from build123d import *

# Parameters (mm, degrees)
F0_R     = 77.1800342887
F0_R_2   = 66.4755295027
F1_DEPTH = 25.4
F2_DEPTH = 25.4
F3_DEPTH = 67.056


with BuildPart() as f1:
    # F0 (on Top) → F1 (new body)
    with BuildSketch(Plane.XY):
        Circle(F0_R)
        Circle(F0_R_2, mode=Mode.SUBTRACT)
    extrude(amount=F1_DEPTH)

    # F2 (add): faces of the model
    f2_faces = [f1.faces().sort_by_distance(p)[0] for p in [
        (-74.997053264, 0, 0),
        (-74.997053264, 0, 25.4),
    ]]
    extrude(f2_faces, amount=F2_DEPTH, dir=(0, 0, -1))

    # F3 (add): a face of the model
    f3_faces = [f1.faces().sort_by_distance(p)[0] for p in [
        (-74.997053264, 0, 25.4),
    ]]
    extrude(f3_faces, amount=F3_DEPTH)


solid = f1.part
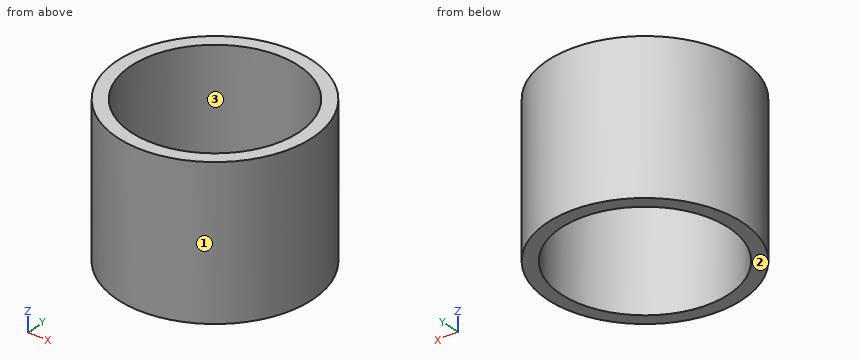
Design review of the part built by this model. Coordinates are the model's own, in mm. Face numbers are marked on the shaded views. Coordinates: 2 decimals unless noted, no trailing zeros. Order: outer loops, then holes, each group sorted by start corner. A loop starts at its lowest first (then second) coordinate and runs counter-clockwise, first axis right, second up. Notation, with made-up numbers: M 74,-4 L 103,-4 A23 ccw 103,30 Z; hole C 13,58.25 d3. An arc over 180 degrees is marked long. Use a Markdown table: item, result.
(1) Wall thickness on probe 1 along Y at (x, z) = (0, 41); probe 2 along X at (y, z) = (-36, -5.5); probe 3 along Y at (x, z) = (41, 76.5): over which ranges is each line inside the solid? List them lowest first.
Worked answers:
| item | result |
|---|---|
| probe 1 | y = -77.18 to -66.48, 66.48 to 77.18 |
| probe 2 | x = -68.27 to -55.88, 55.88 to 68.27 |
| probe 3 | y = -65.39 to -52.33, 52.33 to 65.39 |
(2) Draft analysis for pull direction X (two halves, no side actions). For the marked faces 1, 2 and 3, state which applies: released by +X, released by -X, zero draft, split by the parting line, or undercut.
Worked answers:
| item | result |
|---|---|
| face 1 | split by the parting line |
| face 2 | zero draft |
| face 3 | undercut |
(3) Add section C-C (z = 61.5). Give the boundary of the cut face in (x, y).
Worked answers:
| item | result |
|---|---|
| outline | C 0,0 d154.36; hole C 0,0 d132.95 |
(4) Add section A-A (y = 0). Give the boundary of the cut face in (x, z).
Worked answers:
| item | result |
|---|---|
| outline | M -77.18,-25.4 L -66.48,-25.4 L -66.48,92.46 L -77.18,92.46 Z; M 66.48,-25.4 L 77.18,-25.4 L 77.18,92.46 L 66.48,92.46 Z |
(5) For P1, Ø5, axis at x = -43.5, z = 30.5, coming from the -Y side; P2, Ø2, axis at y = -57.5, z = 3.5, coming from the -X side; P3, Ø3, axis at x = 22, z = 51.5, coming from the +Y side, all flat-tipped, find the tip position at first contact; note any pin that passes through.
Worked answers:
| item | result |
|---|---|
| P1 | stops at y = -65.39 |
| P2 | stops at x = -52.58 |
| P3 | stops at y = 74.41 |
